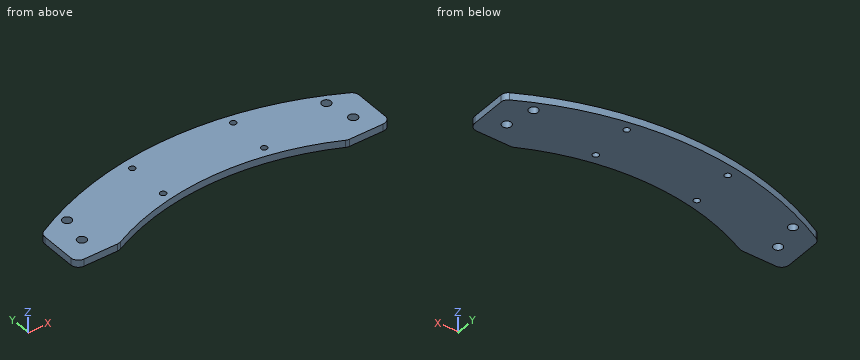
from build123d import *

# Parameters (mm, degrees)
SKETCH1_R           = 2
SKETCH1_R_2         = 3
BOSS_EXTRUDE1_DEPTH = 4.7625


with BuildPart() as part:
    # Sketch1 → Boss-Extrude1 (new body)
    with BuildSketch(Plane.XY):
        with BuildLine():
            Line((-14.25, -9.25), (-14.25, 13.816035512))
            ThreePointArc((-14.25, 13.816035512), (-13.540423999, 16.383575561), (-11.613095238, 18.222369691))
            ThreePointArc((-11.613095238, 18.222369691), (90, 43.75), (191.613095238, 18.222369691))
            ThreePointArc((191.613095238, 18.222369691), (193.540423999, 16.383575561), (194.25, 13.816035512))
            Line((194.25, 13.816035512), (194.25, -9.25))
            ThreePointArc((194.25, -9.25), (192.785533906, -12.785533906), (189.25, -14.25))
            Line((189.25, -14.25), (166.91656424, -14.25))
            ThreePointArc((166.91656424, -14.25), (165.788685845, -14.121128239), (164.718948119, -13.74115613))
            ThreePointArc((164.718948119, -13.74115613), (90, 3.55953545), (15.281051881, -13.74115613))
            ThreePointArc((15.281051881, -13.74115613), (14.211314155, -14.121128239), (13.08343576, -14.25))
            Line((13.08343576, -14.25), (-9.25, -14.25))
            ThreePointArc((-9.25, -14.25), (-12.785533906, -12.785533906), (-14.25, -9.25))
        make_face()
        with Locations((59, 34.290496826)):
            Circle(SKETCH1_R, mode=Mode.SUBTRACT)
        with Locations((59, 6.790496826)):
            Circle(SKETCH1_R, mode=Mode.SUBTRACT)
        with Locations((126, 34.290496826)):
            Circle(SKETCH1_R, mode=Mode.SUBTRACT)
        with Locations((126, 6.790496826)):
            Circle(SKETCH1_R, mode=Mode.SUBTRACT)
        with Locations((180, 0)):
            Circle(SKETCH1_R_2, mode=Mode.SUBTRACT)
        Circle(SKETCH1_R_2, mode=Mode.SUBTRACT)
        with Locations((4, 18.5)):
            Circle(SKETCH1_R_2, mode=Mode.SUBTRACT)
        with Locations((176, 18.5)):
            Circle(SKETCH1_R_2, mode=Mode.SUBTRACT)
    extrude(amount=BOSS_EXTRUDE1_DEPTH)


solid = part.part
Part model, mm, in its own coordinate system. Coordinates: 2 decimals unless noted, no trailing zeros. Loops run counter-clockwise (first coordinate to the right, second up) from the corner with the lowest first, then second, coordinate; pieces in that order, holes last. Notation, with made-up numbers: (79, -10.5) - (135, -10.5) arc R11 cw to (135, -2.5) - close; hole circle Ø2 at (61, 79). An arc over 180 degrees is marked (long way). Write each question's results on one line, items separated by ' | '. Start each with the question number.
Q1. Slice it at A-A on x = 126. Give the cut face in (y, z).
Q2. Slice it at D-D on y = 27.5. Give the cut face in (x, z).
Q3. Slice it at C-C on x = 59. Give the cut face in (y, z).
Q4. Slice it at B-B on z = 2.5. Give the number of separate pieces and of enclosed holes in the cut face, and give its area (3 significant figures).
Q5. Probe line 1 along X through (y, z) = (17, 1.95); line 2 along Y through (x, z) = (59, 2.3); line 3 along Y through (x, z) = (177.5, 2.8). List the from-to ranges inside material, lowest first.
Answer:
1) outline: (-0.3, 0) - (4.79, 0) - (4.79, 4.76) - (-0.3, 4.76) - close; (8.79, 0) - (32.29, 0) - (32.29, 4.76) - (8.79, 4.76) - close; (36.29, 0) - (40.71, 0) - (40.71, 4.76) - (36.29, 4.76) - close
2) outline: (8, 0) - (172, 0) - (172, 4.76) - (8, 4.76) - close
3) outline: (0.71, 0) - (4.79, 0) - (4.79, 4.76) - (0.71, 4.76) - close; (8.79, 0) - (32.29, 0) - (32.29, 4.76) - (8.79, 4.76) - close; (36.29, 0) - (41.5, 0) - (41.5, 4.76) - (36.29, 4.76) - close
4) separate pieces: 1 | enclosed holes: 8 | area: 8,270 mm2
5) line 1: x = -13.11 to 1.4, 6.6 to 173.4, 178.6 to 193.11 | line 2: y = 0.71 to 4.79, 8.79 to 32.29, 36.29 to 41.5 | line 3: y = -14.25 to -1.66, 1.66 to 15.9, 21.1 to 25.14
